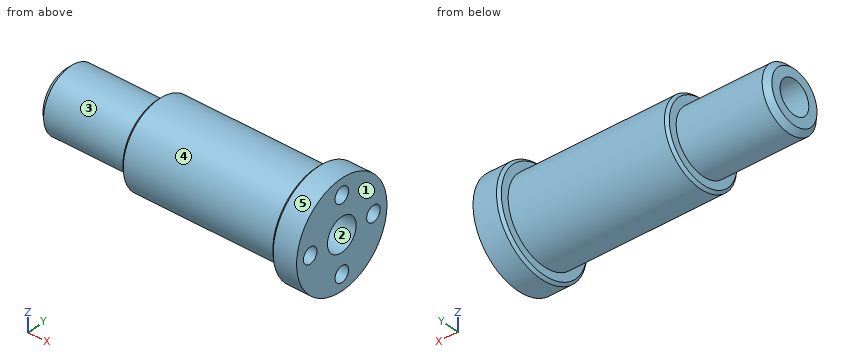
Autodesk Inventor part; units mm, degrees
ref_plane "YZ Plane" through (0, 0, 0) normal (1, 0, 0) x (0, 1, 0)
ref_plane "XZ Plane" through (0, 0, 0) normal (0, 1, 0) x (-1, 0, 0)
ref_plane "XY Plane" through (0, 0, 0) normal (0, 0, 1) x (1, 0, 0)
sketch "Sketch1" plane through (0, 0, 0) normal (0, 0, 1) x (1, 0, 0)
  line L0 (0, 0) -> (0, 10)
  line L1 (0, 10) -> (-5, 10)
  line L2 (-5, 10) -> (-5, 8)
  line L3 (-5, 8) -> (-35.5, 8)
  line L4 (-35.5, 8) -> (-35.5, 6)
  line L5 (-35.5, 6) -> (-53, 6)
  line L6 (-53, 6) -> (-53, 0)
  line L7 (-53, 0) -> (0, 0)
  dimension "d1" = 10
  dimension "d2" = 5
  dimension "d3" = 2
  dimension "d4" = 2
  dimension "d5" = 35.5
  dimension "d6" = 53
revolve "Revolution1" add sketch "Sketch1" angle 360 about axis through (-53, 0, 0) along (1, 0, 0)
thread "Thread1"
chamfer "Chamfer1" distance 1 angle 45 1 edges at (-53, -6, 0)
chamfer "Chamfer2" distance 0.5 angle 45 2 edges at (-35.5, -8, 0) (-5, -10, 0)
sketch "Sketch2" plane through (0, 0, 0) normal (1, 0, 0) x (0, 0, -1)
  circle A0 centre (0, 0) radius 7
  dimension "d17" = 14
hole "Hole1" at (0, 0, 0) direction (-1, 0, 0) diameter 6.35 end through all
sketch "Sketch3" plane through (0, 0, 0) normal (1, 0, 0) x (0, 0, -1)
  circle A0 centre (0, 0) radius 7
  line L0 (0, 0) -> (-7, 0)
  dimension "d25" = 14
hole "Hole2" at (0, 0, 7) direction (-1, 0, 0) diameter 3 depth 4.5 tip angle 118
pattern_circular "Circular Pattern1" count 4 over 360 about axis through (-60.075, 0, 0) along (1, 0, 0) of "Hole2"
properties part number "BronzeHollowScrew" material "Bronze, Soft Tin"
Geometry check sheet. Reference: the model listing, model coordinates, mm. Face numbers are marked on the shaded views. A direction names the side the tool comes from. Round coordinates to 2 decimals unless told otherwise and drop trailing zeros. Order: outer loops, then holes, each group sorted by start corner. A loop starts at its lowest first (then second) coordinate and runs counter-clockwise, first axis right, second up. Notation, with made-up numbers: (-18, 20.25) -> (32, 20.25) arc R22 ccw to (32, 56.25) -> close; hole circle Ø10 at (41, 78). An arc over 180 degrees is marked (long way). Return JSON: item names as keys, results as strings. Group by question number.
Q1. Material ranges on probe 1 along Z at (x, y) = (-28, 0) (3 decimals); probe 2 along Y at (x, z) = (-37.5, 0.25); probe 3 along X at (y, z) = (4, -6.25), recorded low to high. Write a range as from..to.
Q2. Section check A-A, the plane x = -17. Record the boundary of the cut face in (y, z) (3 decimals), plus the area to 3 significant figures.
Q3. Gauge pin test, flat ends, axial feed: pin 1 (1.5 mm diameter, centred on x = -18, z = -3.5, fed in from +Y); pin 2 (4 mm diameter, centred on y = 0, z = 0, fed in from -X); pin 3 (6 mm diameter, centred on x = -18.5, y = -3.5, fed in from +Z); pin 4 (4 mm diameter, centred on x = -11.5, y = -4, fed in from +Z). Record the tip position at first contact, or that the pin passes through.
Q4. Release check for a two-part mould opening along Z. For the marked faces 1, 2 and 3 record: released by +Z, released by -Z, zero draft, split by the parting line, or undercut.
Q5. Tool access check on the marked faces 4 and 5. Record the directions out of +Z, -Z, +X, -X, +Y, -Y that give a thin tool (end or side, any length) a straight path to the whole face; none if there is none.
Numbers:
{
 "1": {"probe 1": "-8..-3.175, 3.175..8", "probe 2": "-5.99..-3.17, 3.17..5.99", "probe 3": "-35.5..0"},
 "2": {"outline": "circle Ø16 at (0, 0); hole circle Ø6.35 at (0, 0)", "area": "169 mm^2"},
 "3": {"pin 1": "y = 7.51", "pin 2": "through", "pin 3": "z = 7.98", "pin 4": "z = 7.75"},
 "4": {"face 1": "zero draft", "face 2": "undercut", "face 3": "split by the parting line"},
 "5": {"face 4": "-X", "face 5": "+X, -X"}
}
